Here's how the part is built. I have some questions about the finished solid (model axes, mm). A direction names the side the tool comes from. Coordinates: 2 decimals unless noted, no trailing zeros. Loops run counter-clockwise (first coordinate to the right, second up) from the corner with the lowest first, then second, coordinate; pieces in that order, holes last.
from build123d import *

# Parameters (mm, degrees)
F0_W     = 75
F0_H     = 75
F0_W_2   = 10
F0_H_2   = 10
F1_DEPTH = 6
F3_DEPTH = 2.75
F5_DEPTH = 2.75


# Not quite as in the source:
# - a feature names something its author has since deleted; it is built from what else it names


with BuildPart() as f1:
    # F0 (on Front) → F1 (new body)
    with BuildSketch(Plane.XZ):
        Rectangle(F0_W, F0_H)
        Rectangle(F0_W_2, F0_H_2, mode=Mode.SUBTRACT)
    extrude(amount=F1_DEPTH)

    # F2 (on face) → F3 (cut)
    with BuildSketch(Plane.XZ.offset(6)):
        Polygon((-24, -19.5), (-2, -19.5), (-2, -5), (-5, -5), (-5, 5), (-2, 5), (-2, 19.5), (-24, 19.5), align=None)
        Polygon((2, -19.5), (24, -19.5), (24, 19.5), (2, 19.5), (2, 5), (5, 5), (5, -5), (2, -5), align=None)
    extrude(amount=-F3_DEPTH, mode=Mode.SUBTRACT)

    # F4 (on face) → F5 (cut)
    with BuildSketch(Plane(origin=(0, 0, 0), x_dir=(-1, 0, 0), z_dir=(0, 1, 0))):
        Polygon((-19.5, -24), (19.5, -24), (19.5, -2.5302600116), (5, -2.5302600116), (5, -5), (-5, -5), (-5, -2.5302600116), (-19.5, -2.5302600116), align=None)
        Polygon((5, 2.5302600116), (19.5, 2.5302600116), (19.5, 24), (-19.5, 24), (-19.5, 2.5302600116), (-5, 2.5302600116), (-5, 5), (5, 5), align=None)
    extrude(amount=-F5_DEPTH, mode=Mode.SUBTRACT)


solid = f1.part
Q1. Will these pins go through, and if not, where does the flat tip stop? P1, Ø6.5, axis at x = -9, z = -7.5, coming from the -Y side; P2, Ø6.5, axis at x = -7.5, z = -11.5, coming from the +Y side.
Q2. We'd pull the mould along Z, two halves only. Please class faces 4 (the flat face through (-12, -1, 2.53)), 5 (the flat face through (8, 0, 1)), 6 (the flat face through (-1, -3, -37.5)), 7 (the flat face through (24, -5, 0)): pulls with the +Z half, pulls with the -Z half, needs draft (parallel to the pull), parting line crosses it, or undercut.
Q3. Suppose I cut it at C-C on z = -17. Write out the boundary of the cut face in (x, y), and give its area (3 significant figures).
Q4. Suppose I cut it at B-B on x = -14.5. Write out the boundary of the cut face in (y, z), and give its area (3 significant figures).
Q5. Suppose I cut it at A-A on y = -1.45. Write out the boundary of the cut face in (x, z), and give its area (3 significant figures).
Q6. Please list where these lines run through material, in increasing order: probe 1 along Z at (x, y) = (-16, -2.15); probe 2 along X at (y, z) = (-5.15, 19); probe 3 along X at (y, z) = (-1.75, -19.5).
Q7. For faces 1 (the flat face through (-13, -5, 19.5)), 2 (the flat face through (0, -4, 5)), 3 (the flat face through (12, -1, -2.53)), which set-ups out of +Z, -Z, +X, -X, +Y, -Y let a thin tool reach every point of the face, with its end or its side?
Check values:
1. P1: stops at y = -3.25
1. P2: stops at y = -2.75
2. face 4: undercut
2. face 5: needs draft
2. face 6: pulls with the -Z half
2. face 7: undercut
3. outline: (-37.5, -6) - (-24, -6) - (-24, -3.25) - (-2, -3.25) - (-2, -6) - (2, -6) - (2, -3.25) - (24, -3.25) - (24, -6) - (37.5, -6) - (37.5, 0) - (19.5, 0) - (19.5, -2.75) - (-19.5, -2.75) - (-19.5, 0) - (-37.5, 0) - close
3. area: 222 mm2
4. outline: (-6, -37.5) - (0, -37.5) - (0, -24) - (-2.75, -24) - (-2.75, -2.53) - (0, -2.53) - (0, 2.53) - (-2.75, 2.53) - (-2.75, 24) - (0, 24) - (0, 37.5) - (-6, 37.5) - (-6, 19.5) - (-3.25, 19.5) - (-3.25, -19.5) - (-6, -19.5) - close
4. area: 225 mm2
5. outline: (-37.5, -37.5) - (37.5, -37.5) - (37.5, 37.5) - (-37.5, 37.5) - close; hole (-19.5, -24) - (19.5, -24) - (19.5, -2.53) - (5, -2.53) - (5, 2.53) - (19.5, 2.53) - (19.5, 24) - (-19.5, 24) - (-19.5, 2.53) - (-5, 2.53) - (-5, -2.53) - (-19.5, -2.53) - close
5. area: 3,900 mm2
6. probe 1: z = -37.5 to -24, -2.53 to 2.53, 24 to 37.5
6. probe 2: x = -37.5 to -24, -2 to 2, 24 to 37.5
6. probe 3: x = -37.5 to -19.5, 19.5 to 37.5
7. face 1: -Y
7. face 2: +Y, -Y
7. face 3: +Y
